Model file for the job. Use its own axes, mm. A direction names the side the tool comes from. Round coordinates to 2 decimals unless told otherwise and drop trailing zeros. Loops run counter-clockwise (first coordinate to the right, second up) from the corner with the lowest first, then second, coordinate; pieces in that order, holes last. Notation, with made-up numbers: M 28,8.5 L 48,8.5 A8 ccw 48,12.5 Z; hole C 50.25,-3 d7. An arc over 180 degrees is marked long. Answer in a Markdown table with one row per item.
from build123d import *

# Parameters (mm, degrees)
AUFSATZ_LINEAR_AUSTRAGEN1_DEPTH = 20


with BuildPart() as part:
    # Skizze1 → Aufsatz-Linear austragen1 (new body)
    with BuildSketch(Plane.XY):
        with BuildLine():
            ThreePointArc((32.5, -10.246334318), (41.488350442, 7.993009877), (32.5, 26.232354072))
            Line((32.5, 26.232354072), (32.5, 35))
            Line((32.5, 35), (15.409785503, 35))
            Line((15.409785503, 35), (7.828556273, 27.418770769))
            ThreePointArc((7.828556273, 27.41877077), (2.44835133, 27.166868372), (1.69484812, 32.5))
            Line((1.69484812, 32.5), (-1.69484812, 32.5))
            ThreePointArc((-1.69484812, 32.5), (-2.44835133, 27.166868372), (-7.828556273, 27.41877077))
            Line((-7.828556273, 27.418770769), (-15.409785503, 35))
            Line((-15.409785503, 35), (-32.5, 35))
            Line((-32.5, 35), (-32.5, 26.232354072))
            ThreePointArc((-32.5, 26.232354072), (-41.488350442, 7.993009877), (-32.5, -10.246334318))
            Line((-32.5, -10.246334318), (-32.5, -35))
            Line((-32.5, -35), (32.5, -35))
            Line((32.5, -35), (32.5, -10.246334318))
        make_face()
        with BuildLine():
            Line((30, 32.5), (30, 24.955672535))
            ThreePointArc((30, 24.955672535), (38.988350442, 7.993009877), (30, -8.969652782))
            Line((30, -8.969652782), (30, -32.5))
            Line((30, -32.5), (-30, -32.5))
            Line((-30, -32.5), (-30, -8.969652782))
            ThreePointArc((-30, -8.969652782), (-38.988350442, 7.993009877), (-30, 24.955672535))
            Line((-30, 24.955672535), (-30, 32.5))
            Line((-30, 32.5), (-15.031105847, 32.5))
            Line((-15.031105847, 32.5), (-8.889216445, 26.358110598))
            ThreePointArc((-8.889216445, 26.358110598), (-4.026954213, 24.833979762), (0, 27.956191892))
            ThreePointArc((0, 27.956191892), (4.026954213, 24.833979762), (8.889216445, 26.358110598))
            Line((8.889216445, 26.358110598), (15.031105847, 32.5))
            Line((15.031105847, 32.5), (30, 32.5))
        make_face(mode=Mode.SUBTRACT)
    extrude(amount=AUFSATZ_LINEAR_AUSTRAGEN1_DEPTH)


solid = part.part
1. Pin check, flat tips, straight feed: pin 1 (1 mm diameter, centred on x = -10.5, z = 8, fed in from +Y); pin 2 (4 mm diameter, centred on y = 29, z = 7, fed in from -X); pin 3 (3 mm diameter, centred on y = 14.5, z = 16.5, fed in from +X). Stop position of each tip, or through.
Verdict:
| item | result |
|---|---|
| pin 1 | stops at y = 30.59 |
| pin 2 | stops at x = -32.5 |
| pin 3 | stops at x = 40.94 |
2. Saw through at C-C (z = 7.5). Write the cut outline in (x, y), and give its area (3 significant figures).
Verdict:
| item | result |
|---|---|
| outline | M -32.5,-35 L 32.5,-35 L 32.5,-10.25 A23 ccw 32.5,26.23 L 32.5,35 L 15.41,35 L 7.83,27.42 A4 cw 1.69,32.5 L -1.69,32.5 A4 cw -7.83,27.42 L -15.41,35 L -32.5,35 L -32.5,26.23 A23 ccw -32.5,-10.25 Z; hole M -30,-32.5 L 30,-32.5 L 30,-8.97 A20.5 ccw 30,24.96 L 30,32.5 L 15.03,32.5 L 8.89,26.36 A5.5 cw 0,27.96 A5.5 cw -8.89,26.36 L -15.03,32.5 L -30,32.5 L -30,24.96 A20.5 ccw -30,-8.97 Z |
| area | 670 mm² |
3. Saw through at A-A (y = -17). Write the cut outline in (x, z).
Verdict:
| item | result |
|---|---|
| outline | M -32.5,0 L -30,0 L -30,20 L -32.5,20 Z; M 30,0 L 32.5,0 L 32.5,20 L 30,20 Z |
4. Tool access for faces 1 (the flat face through (0, 32.5, 10)), 2 (the flat face through (-32.5, -22, 10)), 3 (the flat face through (11.92, 29.39, 9.86)), 4 (the cylindrical face through (41.486, 7.698, 9.86)), 5 (the flat face through (-3, 26, 20)): list every direction of +Z, -Z, +X, -X, +Y, -Y with a clear straight run to the whole face (end or side of a thin tool).
Verdict:
| item | result |
|---|---|
| face 1 | +Z, -Z, +Y |
| face 2 | +Z, -Z, -X, -Y |
| face 3 | +Z, -Z |
| face 4 | +Z, -Z, +X |
| face 5 | +Z, +X, -X, +Y, -Y |
5. Wall check: probe 1 along Y at (x, z) = (-25, 10); probe 2 along X at (y, z) = (-18, 10.5); probe 3 along X at (y, z) = (31, 7). Give the ranges that are in metal, low to high.
Verdict:
| item | result |
|---|---|
| probe 1 | y = -35 to -32.5, 32.5 to 35 |
| probe 2 | x = -32.5 to -30, 30 to 32.5 |
| probe 3 | x = -32.5 to -30, -13.53 to -11.41, -1.07 to 1.07, 11.41 to 13.53, 30 to 32.5 |
6. Saw through at B-B (x = -5). Write the cut outline in (y, z), and give its area (3 significant figures).
Verdict:
| item | result |
|---|---|
| outline | M -35,0 L -32.5,0 L -32.5,20 L -35,20 Z; M 24.75,0 L 26.25,0 L 26.25,20 L 24.75,20 Z |
| area | 80.0 mm² |
7. Mould opens along X. For faces 6 (the flat face through (22, 32.5, 10)), 7 (the flat face through (-32.5, 31, 10)), 8 (the flat face through (0, -35, 10)) say: +X half, -X half, draft (parallel to the pull), parting line (faces both ways), or undercut.
Verdict:
| item | result |
|---|---|
| face 6 | undercut |
| face 7 | -X half |
| face 8 | draft |
